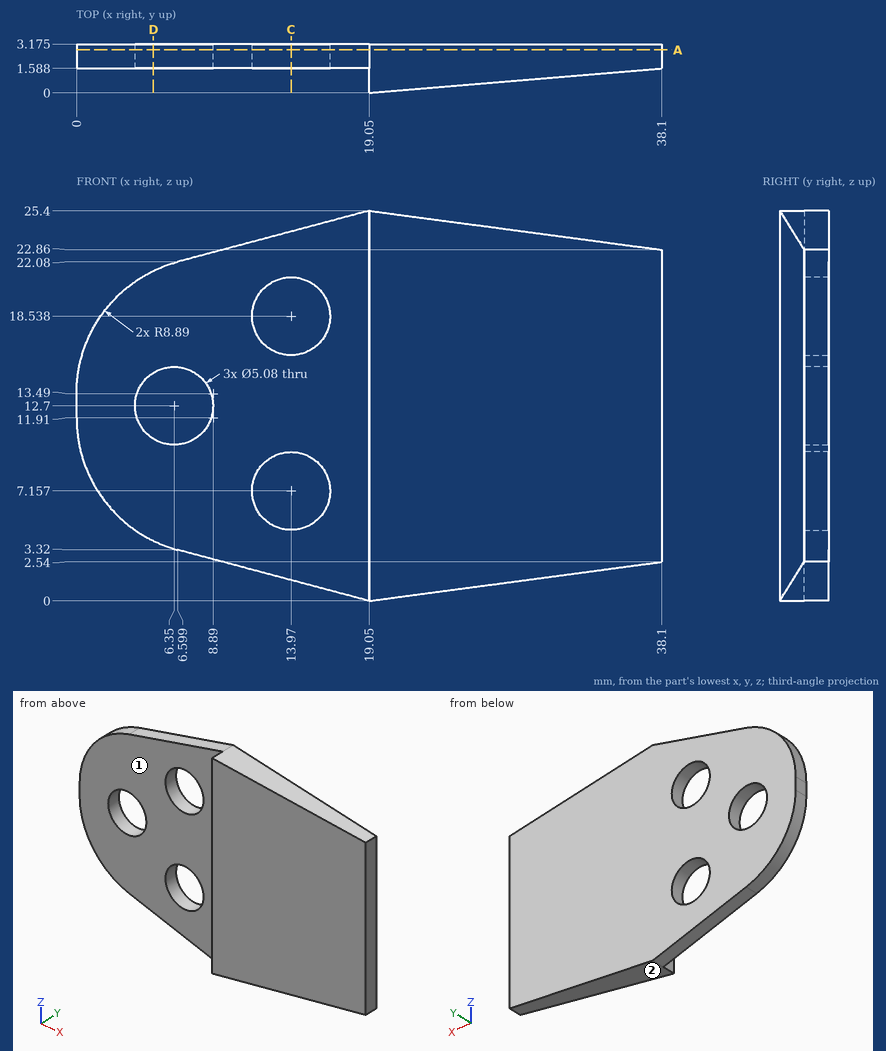
The drawing under review shows one solid part. Ordinate dimensions are in mm from its lowest x, y, z. A direction names the side the tool comes from. Round coordinates to 2 decimals unless told otherwise and drop trailing zeros. Order: outer loops, then holes, each group sorted by start corner. A loop starts at its lowest first (then second) coordinate and runs counter-clockwise, first axis right, second up. Notation, with made-up numbers: (-12.75, 76.5) - (5.25, 76.5) arc R33 ccw to (5.25, 112.5) - close; hole circle Ø7 at (34.25, 73.25). An arc over 180 degrees is marked (long way). Return JSON: item names as keys, results as strings.
Q1. Consider section D-D on x = 5. Write out the cut boundary in (y, z) (1 decimal).
Computed values:
{"outline": "(1.6, 3.9) - (3.2, 3.9) - (3.2, 10.5) - (1.6, 10.5) - close; (1.6, 14.9) - (3.2, 14.9) - (3.2, 21.5) - (1.6, 21.5) - close"}
Q2. Consider section A-A on y = 2.8. Write out the cut boundary in (x, z).
Computed values:
{"outline": "(0, 11.91) arc R8.89 ccw to (6.6, 3.32) - (19.05, 0) - (38.1, 2.54) - (38.1, 22.86) - (19.05, 25.4) - (6.6, 22.08) arc R8.89 ccw to (0, 13.49) - close; hole circle Ø5.08 at (6.35, 12.7); hole circle Ø5.08 at (13.97, 7.16); hole circle Ø5.08 at (13.97, 18.54)"}
Q3. For pin 1 Ø15 at (x, z) = (5, 9.5) entering from -Y; pin 2 Ø4.5 at (x, z) = (13.97, 7.16) entering from +Y; pin 3 Ø0.5 at (y, z) = (0.5, 14.5) entering from -X; pin 4 Ø5 at (x, z) = (28, 19.5) entering from -Y, all flat-tipped, find the tip position at first contact; note any pin that passes through.
Computed values:
{"pin 1": "stops at y = 1.59", "pin 2": "passes through", "pin 3": "stops at x = 19.05", "pin 4": "stops at y = 0.54"}
Q4. Wall thickness on L1, parallel to X at y = 2.7, z = 12.7; L2, parallel to Z at x = 14.5, y = 2.5 (1 decimal); L3, parallel to Y at x = 2, z = 10.5 (1 decimal): over which ranges is each line inside the solid? List them lowest first. Write a range as [from, to].
Computed values:
{"L1": "x = [0, 3.81], [8.89, 38.1]", "L2": "z = [1.2, 4.7], [9.6, 16.1], [21, 24.2]", "L3": "y = [1.6, 3.2]"}
Q5. Consider section C-C on x = 13.97. Write out the cut boundary in (y, z) (1 decimal).
Computed values:
{"outline": "(1.6, 1.4) - (3.2, 1.4) - (3.2, 4.6) - (1.6, 4.6) - close; (1.6, 9.7) - (3.2, 9.7) - (3.2, 16) - (1.6, 16) - close; (1.6, 21.1) - (3.2, 21.1) - (3.2, 24) - (1.6, 24) - close"}
Q6. Machinability: for the marked faces 1 and 2, which of the approach directions +Z, -Z, +X, -X, +Y, -Y give a long, thin tool a straight path to every point of the face, cutting with its end or side? Answer none if there is none.
Computed values:
{"face 1": "+Z, -Z, -X, -Y", "face 2": "-Z, +X, +Y, -Y"}
